The model under review builds one solid part; all positions refer to its coordinate system, in mm. Face numbers are marked on the shaded views. Round coordinates to 2 decimals unless told otherwise and drop trailing zeros. Order: outer loops, then holes, each group sorted by start corner. A loop starts at its lowest first (then second) coordinate and runs counter-clockwise, first axis right, second up.
```python
from build123d import *

# Parameters (mm, degrees)
SKETCH1_W           = 118
SKETCH1_H           = 111
SKETCH1_W_2         = 100
SKETCH1_H_2         = 93
BOSS_EXTRUDE1_DEPTH = 9
SKETCH2_W           = 100
SKETCH2_H           = 93
SKETCH2_R           = 3.175
CUT_EXTRUDE1_DEPTH  = 5
SKETCH2_3_R         = 3.175
CUT_EXTRUDE2_DEPTH  = 115.906483716


with BuildPart() as part:
    # Sketch1 → Boss-Extrude1 (new body)
    # profile 1 of 6: a face of its own
    with BuildSketch(Plane(origin=(0, 0, 0), x_dir=(1, 0, 0), z_dir=(0, 1, 0))):
        Rectangle(SKETCH1_W, SKETCH1_H)
        Rectangle(SKETCH1_W_2, SKETCH1_H_2, mode=Mode.SUBTRACT)
    # profile 2 of 6: a face of its own
    with BuildSketch(Plane(origin=(0, 0, 0), x_dir=(1, 0, 0), z_dir=(0, 1, 0))):
        Rectangle(SKETCH1_W_2, SKETCH1_H_2)
    # profile 3 of 6: a face of its own
    with BuildSketch(Plane(origin=(0, 0, 0), x_dir=(1, 0, 0), z_dir=(0, 1, 0))):
        with BuildLine():
            Line((-59, -55.5), (-59, 55.5))
            ThreePointArc((-59, 55.5), (-81.001543195, 0), (-59, -55.5))
        make_face()
    # profile 4 of 6: a face of its own
    with BuildSketch(Plane(origin=(0, 0, 0), x_dir=(1, 0, 0), z_dir=(0, 1, 0))):
        with BuildLine():
            Line((59, -55.5), (-59, -55.5))
            ThreePointArc((-59, -55.5), (0, -81.001543195), (59, -55.5))
        make_face()
    # profile 5 of 6: a face of its own
    with BuildSketch(Plane(origin=(0, 0, 0), x_dir=(1, 0, 0), z_dir=(0, 1, 0))):
        with BuildLine():
            ThreePointArc((81.001543195, 0), (75.300534688, 29.850954352), (59, 55.5))
            Line((59, 55.5), (59, -55.5))
            ThreePointArc((59, -55.5), (75.300534688, -29.850954352), (81.001543195, 0))
        make_face()
    # profile 6 of 6: a face of its own
    with BuildSketch(Plane(origin=(0, 0, 0), x_dir=(1, 0, 0), z_dir=(0, 1, 0))):
        with BuildLine():
            ThreePointArc((59, 55.5), (0, 81.001543195), (-59, 55.5))
            Line((-59, 55.5), (59, 55.5))
        make_face()
    extrude(amount=BOSS_EXTRUDE1_DEPTH)

    # Sketch2 → Cut-Extrude1 (cut)
    with BuildSketch(Plane(origin=(0, 9, 0), x_dir=(1, 0, 0), z_dir=(0, 1, 0))):
        Rectangle(SKETCH2_W, SKETCH2_H)
        with Locations(Location((-24.919571738, -23.175201717, 0), (0, 0, 270))):
            Circle(SKETCH2_R, mode=Mode.SUBTRACT)
        with Locations(Location((24.919571738, -23.175201717, 0), (0, 0, 270))):
            Circle(SKETCH2_R, mode=Mode.SUBTRACT)
        with Locations(Location((24.919571738, 23.175201717, 0), (0, 0, 270))):
            Circle(SKETCH2_R, mode=Mode.SUBTRACT)
        with Locations(Location((-24.919571738, 23.175201717, 0), (0, 0, 270))):
            Circle(SKETCH2_R, mode=Mode.SUBTRACT)
    extrude(amount=-CUT_EXTRUDE1_DEPTH, mode=Mode.SUBTRACT)

    # Sketch2_3 → Cut-Extrude2 (cut, through all)
    with BuildSketch(Plane(origin=(0, 9, 0), x_dir=(1, 0, 0), z_dir=(0, 1, 0))):
        with Locations(Location((-24.919571738, -23.175201717, 0), (0, 0, 270))):
            Circle(SKETCH2_3_R)
        with Locations(Location((24.919571738, -23.175201717, 0), (0, 0, 270))):
            Circle(SKETCH2_3_R)
        with Locations(Location((24.919571738, 23.175201717, 0), (0, 0, 270))):
            Circle(SKETCH2_3_R)
        with Locations(Location((-24.919571738, 23.175201717, 0), (0, 0, 270))):
            Circle(SKETCH2_3_R)
    extrude(amount=-CUT_EXTRUDE2_DEPTH, mode=Mode.SUBTRACT)


solid = part.part
```
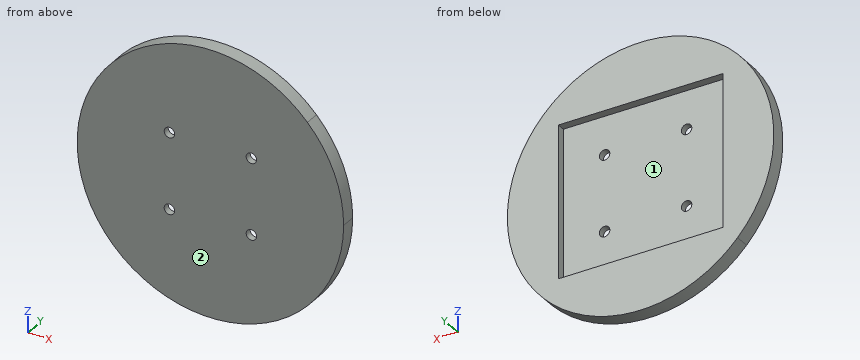
(1) Insertion check: pin 1 (4 mm diameter, centred on y = 7.5, z = -17.5, fed in from -X); pin 2 (3 mm diameter, centred on y = 2.5, z = 15, fed in from +X); pin 3 (7.5 mm diameter, centred on x = 24.92, z = -23.18, fed in from -Y); pin 4 (1 mm diameter, centred on y = 3, z = 34.5, fed in from -X). Each pin has a flat end and moves straight along its axis. Give the tip position at first contact, or say it passes through.
Data:
pin 1: stops at x = -79.5
pin 2: stops at x = 79.87
pin 3: stops at y = 0
pin 4: stops at x = -73.52
(2) Consider section C-C (z = -17). Write out the cut boundary in (x, y).
Data:
outline: (-79.2, 0) - (79.2, 0) - (79.2, 9) - (50, 9) - (50, 4) - (-50, 4) - (-50, 9) - (-79.2, 9) - close
(3) Consider section A-A (y = 6). Write out the cut boundary in (x, z), and give its area (3 significant figures).
Data:
outline: circle Ø162 at (0, 0); hole (-50, -46.5) - (50, -46.5) - (50, 46.5) - (-50, 46.5) - close
area: 11,300 mm2
(4) To check wall thickness, follow probe 1 along X at (y, z) = (0.5, -26); probe 2 along Z at (x, y) = (25.5, 3.5); probe 3 along Z at (x, y) = (-0.5, 1.75). State the ranges of each line that lie inside material, in increasing order.
Data:
probe 1: x = -76.72 to -26.37, -23.47 to 23.47, 26.37 to 76.72
probe 2: z = -76.88 to -26.3, -20.05 to 20.05, 26.3 to 76.88
probe 3: z = -81 to 81
(5) Consider section D-D (z = 61). Write out the cut boundary in (x, y).
Data:
outline: (-53.29, 0) - (53.29, 0) - (53.29, 9) - (-53.29, 9) - close
(6) Consider section B-B (x = -46.5). Write out the cut boundary in (y, z), and give its area (3 significant figures).
Data:
outline: (0, -66.32) - (9, -66.32) - (9, -46.5) - (4, -46.5) - (4, 46.5) - (9, 46.5) - (9, 66.32) - (0, 66.32) - close
area: 729 mm2
(7) Draft analysis for pull direction X (two halves, no side actions). For the marked faces 1 and 2, state which applies: pulls with the +X half, pulls with the -X half, needs draft (parallel to the pull), parting line crosses it, or undercut.
Data:
face 1: undercut
face 2: needs draft
